Part model, mm, in its own coordinate system. A direction names the side the tool comes from. Round coordinates to 2 decimals unless told otherwise and drop trailing zeros. Order: outer loops, then holes, each group sorted by start corner. A loop starts at its lowest first (then second) coordinate and runs counter-clockwise, first axis right, second up. Notation, with made-up numbers: (64, 0) - (77, 0) arc R14 ccw to (77, 13) - close; hole circle Ø5 at (-36, 41). An arc over 180 degrees is marked (long way). Answer as a JSON object with one key per item and string values.
```python
from build123d import *

# Parameters (mm, degrees)
F1_DEPTH = 2000
F2_R     = 5
F3_DEPTH = 3


with BuildPart() as f1:
    # F0 (on Front) → F1 (new body)
    with BuildSketch(Plane.XZ):
        with BuildLine():
            Line((40, 0), (0, 0))
            Line((0, 0), (0, -40))
            Line((0, -40), (3, -40))
            Line((3, -40), (3, -8))
            ThreePointArc((3, -8), (4.464466, -4.464466), (8, -3))
            Line((8, -3), (40, -3))
            Line((40, -3), (40, 0))
        make_face()
    extrude(amount=F1_DEPTH)

    # F2 (on face) → F3 (cut, through all)
    with BuildSketch(Plane(origin=(0, 0, 0), x_dir=(0, -1, 0), z_dir=(-1, 0, 0))):
        with Locations((50, -20)):
            Circle(F2_R)
        with Locations((150, -20)):
            Circle(F2_R)
        with Locations((250, -20)):
            Circle(F2_R)
        with Locations((350, -20)):
            Circle(F2_R)
        with Locations((450, -20)):
            Circle(F2_R)
        with Locations((550, -20)):
            Circle(F2_R)
        with Locations((650, -20)):
            Circle(F2_R)
        with Locations((750, -20)):
            Circle(F2_R)
        with Locations((850, -20)):
            Circle(F2_R)
        with Locations((950, -20)):
            Circle(F2_R)
        with Locations((1050, -20)):
            Circle(F2_R)
        with Locations((1150, -20)):
            Circle(F2_R)
        with Locations((1250, -20)):
            Circle(F2_R)
        with Locations((1350, -20)):
            Circle(F2_R)
        with Locations((1450, -20)):
            Circle(F2_R)
        with Locations((1550, -20)):
            Circle(F2_R)
        with Locations((1650, -20)):
            Circle(F2_R)
        with Locations((1750, -20)):
            Circle(F2_R)
        with Locations((1850, -20)):
            Circle(F2_R)
        with Locations((1950, -20)):
            Circle(F2_R)
        with Locations((2050, -20)):
            Circle(F2_R)
        with Locations((2150, -20)):
            Circle(F2_R)
        with Locations((2250, -20)):
            Circle(F2_R)
        with Locations((2350, -20)):
            Circle(F2_R)
        with Locations((2450, -20)):
            Circle(F2_R)
    extrude(amount=-F3_DEPTH, mode=Mode.SUBTRACT)


solid = f1.part
```
Item 1: Drop flat-ended pins along their axis: P1, Ø1.5, axis at x = 21.5, y = -515.5, coming from the -Z side; P2, Ø12, axis at y = -327, z = -17, coming from the +X side. Give the stop position or say it passes through.
Taken from the geometry:
{"P1": "z = -3", "P2": "x = 3"}
Item 2: Probe L1, parallel to Z at x = 1.4, y = -1950; L2, parallel to X at y = -86, z = -14.5; L3, parallel to Z at x = 25.5, y = -256.5. List the from-to ranges inside material, lowest first. Write a range as from..to.
Taken from the geometry:
{"L1": "-40..-25, -15..0", "L2": "0..3", "L3": "-3..0"}
Item 3: Cut at A-A (x = 15.5). Write the cut outline in (y, z).
Taken from the geometry:
{"outline": "(-2000, -3) - (0, -3) - (0, 0) - (-2000, 0) - close"}
Item 4: Tool access for faces 1 (the flat face through (0, -986, -20)), 2 (the flat face through (3, -986, -24)): list every direction of +Z, -Z, +X, -X, +Y, -Y with a clear straight run to the whole face (end or side of a thin tool).
Taken from the geometry:
{"face 1": "+Z, -Z, -X, +Y, -Y", "face 2": "-Z, +X, +Y, -Y"}
